from build123d import *

# Parameters (mm, degrees)
BOSS_EXTRUDE1_DEPTH = 65
SHELL1_T            = -2
CUT_EXTRUDE1_DEPTH  = 100
FILLET1_R           = 5
SKETCH3_R           = 3.5
CUT_EXTRUDE2_DEPTH  = 100


with BuildPart() as part:
    # Sketch1 → Boss-Extrude1 (new body, symmetric)
    with BuildSketch(Plane(origin=(0, 0, 0), x_dir=(0, 0, -1), z_dir=(1, 0, 0))):
        Polygon((0, 60), (-28.284271247, 31.715728753), (0, 0), (10, 0), (10, 60), align=None)
    extrude(amount=BOSS_EXTRUDE1_DEPTH, both=True)

    # Shell1
    shell1_openings = [part.faces().sort_by_distance(p)[0] for p in [
        (0, 30, -10),
    ]]
    offset(amount=SHELL1_T, openings=shell1_openings, kind=Kind.INTERSECTION)

    # Sketch2 → Cut-Extrude1 (cut)
    with BuildSketch(Plane(origin=(0, 30, 30), x_dir=(1, 0, 0), z_dir=(0, 0.707106781, 0.707106781))):
        with BuildLine():
            Line((15.3, 10.276406871), (-54, 10.276406871))
            ThreePointArc((-54, 10.276406871), (-54.707106781, 10.56930009), (-55, 11.276406871))
            Line((-55, 11.276406871), (-55, 33.576406871))
            ThreePointArc((-55, 33.576406871), (-54.707106781, 34.283513652), (-54, 34.576406871))
            Line((-54, 34.576406871), (15.3, 34.576406871))
            ThreePointArc((15.3, 34.576406871), (16.007106781, 34.283513652), (16.3, 33.576406871))
            Line((16.3, 33.576406871), (16.3, 11.276406871))
            ThreePointArc((16.3, 11.276406871), (16.007106781, 10.56930009), (15.3, 10.276406871))
        make_face()
    extrude(amount=-CUT_EXTRUDE1_DEPTH, mode=Mode.SUBTRACT)

    # Fillet1
    fillet1_edges = [part.edges().sort_by_distance(p)[0] for p in [
        (65, 45.857864376, 14.142135624),
        (65, 15.857864376, 14.142135624),
        (-65, 15.857864376, 14.142135624),
        (-65, 45.857864376, 14.142135624),
        (0, 31.715728753, 28.284271247),
        (0, 60, 0),
    ]]
    fillet(fillet1_edges, radius=FILLET1_R)

    # Sketch3 → Cut-Extrude2 (cut)
    with BuildSketch(Plane(origin=(0, 30, 30), x_dir=(1, 0, 0), z_dir=(0, 0.707106781, 0.707106781))):
        with Locations((38.15, 22.426406871)):
            Circle(SKETCH3_R)
    extrude(amount=-CUT_EXTRUDE2_DEPTH, mode=Mode.SUBTRACT)


solid = part.part
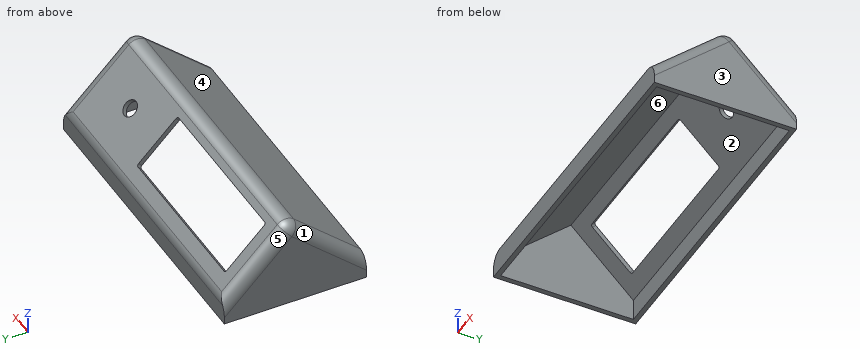
Read the model definition and answer for the solid it produces. Units are mm, in the model's axes. Face numbers are marked on the shaded views. A direction names the side the tool comes from. Round coordinates to 2 decimals unless told otherwise and drop trailing zeros. Order: outer loops, then holes, each group sorted by start corner. A loop starts at its lowest first (then second) coordinate and runs counter-clockwise, first axis right, second up. Notation, with made-up numbers: (-7.75, 38) - (10.25, 38) arc R20 cw to (10.25, 56) - close; hole circle Ø3 at (3.5, 28). An arc over 180 degrees is marked (long way). Use one line per item in the form item = value. Start each with the question number.
(1) The part is cut by section B-B (x = 55.5). Give the vertices of the cut face in (y, z).
(2) Find the intervals of material crossed by line 1 along X through (y, z) = (18, 5); line 2 along Y through (x, z) = (-45, -2); line 3 along Y through (x, z) = (-60, 21), in increasing order. Write a range as from..to.
(3) For the marked faces 1 and 2, determine the directions among +Z, -Z, +X, -X, +Y, -Y from which every point of the face is accessible in a straight line to the end or side of a thin tool.
(4) Flat-ended cylindrical pins translate along their axes: pin 1 Ø1 at (x, y) = (-17.5, 15.5) entering from +Z; pin 2 Ø4 at (x, z) = (-7, 0.5) entering from +Y; pin 3 Ø12 at (x, y) = (20, 53.5) entering from +Z. Find the tip coordinate at first contact, or state that the pin passes through.
(5) The part is cut by section A-A (x = 13.5). Give the vertices of the cut face in (y, z) (3 decimals).
(6) Determine the mould class of the marked faces 3, 4, 5 and 6 for opening direction X: +X half, -X half, draft (parallel to the pull), parting line (faces both ways), or undercut.
Checked values:
q1.outline = (0, -10) - (2, -10) - (2, -0.9) - (31.64, 25.53) - (58, -0.83) - (58, -10) - (60, -10) - (60, -2.07) arc R5 ccw to (58.54, 1.46) - (35.05, 24.95) arc R5 ccw to (28.19, 25.14) - (0, 0) - close
q2.line_1 = -65..-63, 63..65
q2.line_2 = 0..2, 58..60
q2.line_3 = 23.55..26.55, 36.17..39
q3.face_1 = +Z, -X, -Y
q3.face_2 = -Z
q4.pin_1 = 14.27
q4.pin_2 = 59.97
q4.pin_3 = 12.5
q5.outline = (0, -10) - (2, -10) - (2, -0.896) - (31.637, 25.534) - (35.852, 21.319) - (37.267, 22.733) - (35.055, 24.945) arc R5 ccw to (28.191, 25.141) - (0, 0) - close; (53.035, 4.137) - (58, -0.828) - (58, -10) - (60, -10) - (60, -2.071) arc R5 ccw to (58.536, 1.464) - (54.449, 5.551) - close
q6.face_3 = +X half
q6.face_4 = draft
q6.face_5 = -X half
q6.face_6 = undercut
